Check sheet for the modelled part. Datum: model origin and axes. Units: mm. Face numbers are marked on the shaded views. A direction names the side the tool comes from. Give positions to 0.01 mm unless a question says otherwise; leave off trailing zeros. Loops run counter-clockwise (first coordinate to the right, second up) from the corner with the lowest first, then second, coordinate; pieces in that order, holes last. Notation, with made-up numbers: M -10.5,-40 L 48.5,-40 A21 ccw 48.5,-21 Z; hole C 27,29 d4. An arc over 180 degrees is marked long. Write each question's results on one line, items separated by ' | '. Start each with the question number.
1. Tool access check on the marked faces 4 and 5. Record the directions out of +Z, -Z, +X, -X, +Y, -Y that give a thin tool (end or side, any length) a straight path to the whole face; none if there is none.
2. Sectioned sample at D-D on z = 1. Record the cut outline in (x, y).
3. Draft check along Y on the marked faces 1, 2 and 3. Enter one of: pulls with the +Y half, pulls with the -Y half, needs draft (parallel to the pull), parting line crosses it, or undercut.
4. Material ranges on line 1 along X through (y, z) = (0.5, 1.4); line 2 along Y through (x, z) = (0, 2.5); line 3 along Z through (x, y) = (5, -1), recorded low to high.
5. Sectioned sample at B-B on x = 0. Record the cut outline in (y, z), and give its area (3 significant figures).
6. Go/stop test with flat-tipped pins: pin 1 (2 mm diameter, centred on x = -3.5, z = 1, fed in from -Y); pin 2 (1 mm diameter, centred on x = 5.5, y = 0, fed in from -Z). Record where each tip stops, or that it passes through.
7. Sectioned sample at C-C on z = 3.2. Record the cut outline in (x, y), and give its area (3 significant figures).
8. Sectioned sample at A-A on y = 0. Record the cut outline in (x, z), and give its area (3 significant figures).
Autodesk Inventor part; units mm, degrees
ref_plane "YZ Plane" through (0, 0, 0) normal (1, 0, 0) x (0, 1, 0)
ref_plane "XZ Plane" through (0, 0, 0) normal (0, 1, 0) x (-1, 0, 0)
ref_plane "XY Plane" through (0, 0, 0) normal (0, 0, 1) x (1, 0, 0)
sketch "Skizze1" plane through (0, 0, 0) normal (0, 0, 1) x (1, 0, 0)
  circle A0 centre (0, 0) radius 8
  dimension "d0" = 16
extrude "Extrusion1" add sketch "Skizze1" along normal blind 3
sketch "Skizze2" plane through (0, 0, 3) normal (0, 0, 1) x (1, 0, 0)
  circle A0 centre (0, 0) radius 2.5
  dimension "d3" = 5
extrude "Extrusion2" add sketch "Skizze2" along normal blind 1
sketch "Skizze3" plane through (0, 0, 4) normal (0, 0, 1) x (1, 0, 0)
  circle A0 centre (0, 0) radius 2.5
hole "Bohrung1" at (0, 0, 4) direction (0, 0, -1) diameter 3 depth 4
sketch "Skizze4" plane through (0, 0, 3) normal (0, 0, 1) x (1, 0, 0)
  point P0 (0, 0)
  point P1 (5.5, 0)
  dimension "d20" = 5.5
hole "Bohrung2" at (5.5, 0, 3) direction (0, 0, -1) diameter 1.6 end through all
chamfer "Fasen1" distance 0.15 angle 45 1 edges at (-8, 0, 3)
chamfer "Fasen2" distance 0.09 angle 45 1 edges at (-2.5, 0, 4)
properties part number "Kurbel" material "Gold"
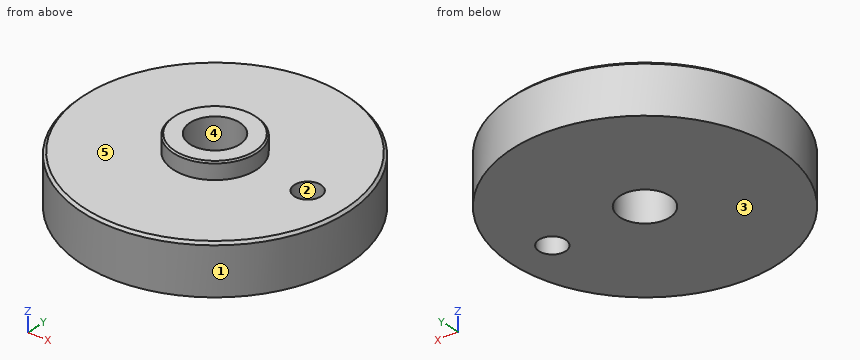
Output values:
1) face 4: +Z, -Z | face 5: +Z
2) outline: C 0,0 d16; hole C 0,0 d3; hole C 5.5,0 d1.6
3) face 1: parting line crosses it | face 2: undercut | face 3: needs draft
4) line 1: -7.98 to -1.41, 1.41 to 4.88, 6.12 to 7.98 | line 2: -8 to -1.5, 1.5 to 8 | line 3: 0 to 3
5) outline: M -8,0 L -1.5,0 L -1.5,4 L -2.41,4 L -2.5,3.91 L -2.5,3 L -7.85,3 L -8,2.85 Z; M 1.5,0 L 8,0 L 8,2.85 L 7.85,3 L 2.5,3 L 2.5,3.91 L 2.41,4 L 1.5,4 Z | area: 41.0 mm2
6) pin 1: y = -7.6 | pin 2: through
7) outline: C 0,0 d5; hole C 0,0 d3 | area: 12.6 mm2
8) outline: M -8,0 L -1.5,0 L -1.5,4 L -2.41,4 L -2.5,3.91 L -2.5,3 L -7.85,3 L -8,2.85 Z; M 1.5,0 L 4.7,0 L 4.7,3 L 2.5,3 L 2.5,3.91 L 2.41,4 L 1.5,4 Z; M 6.3,0 L 8,0 L 8,2.85 L 7.85,3 L 6.3,3 Z | area: 36.2 mm2
